from build123d import *

# Parameters (mm, degrees)
SKETCH1_R               = 18.5
BOSS_EXTRUDE1_DEPTH     = 60
SKETCH2_W               = 40
SKETCH2_H               = 37
BOSS_EXTRUDE2_DEPTH     = 58
SKETCH3_R               = 4
BOSS_EXTRUDE3_DEPTH     = 15
CUT_EXTRUDE1_DEPTH      = 125.282943319
CUT_EXTRUDE1_DEPTH_BACK = 58
SKETCH4_W               = 40
SKETCH4_H               = 10
SKETCH5_R               = 4
SKETCH5_R_2             = 2.25
BOSS_EXTRUDE4_DEPTH     = 1.5


with BuildPart() as part:
    # Sketch1 → Boss-Extrude1 (new body)
    with BuildSketch(Plane.XY):
        Circle(SKETCH1_R)
    extrude(amount=BOSS_EXTRUDE1_DEPTH)

    # Sketch2 → Boss-Extrude2 (add)
    with BuildSketch(Plane.XY.offset(60)):
        Rectangle(SKETCH2_W, SKETCH2_H)
    extrude(amount=BOSS_EXTRUDE2_DEPTH)

    # Sketch3 → Boss-Extrude3 (add)
    with BuildSketch(Plane(origin=(0, 18.5, 0), x_dir=(1, 0, 0), z_dir=(0, 1, 0))):
        with Locations(Location((0, -98, 0), (0, 0, 90))):
            Circle(SKETCH3_R)
    extrude(amount=BOSS_EXTRUDE3_DEPTH)

    # Sketch4 → Cut-Extrude1 (cut, two sides: drawn at the far end of the back side and taken through both)
    with BuildSketch(Plane.XY.offset(118).offset(-CUT_EXTRUDE1_DEPTH_BACK)):
        with Locations((0, -13.5)):
            Rectangle(SKETCH4_W, SKETCH4_H)
    extrude(amount=CUT_EXTRUDE1_DEPTH + CUT_EXTRUDE1_DEPTH_BACK, mode=Mode.SUBTRACT)

    # Sketch5 → Boss-Extrude4 (add)
    # profile 1 of 4: a face of its own
    with BuildSketch(Plane(origin=(0, 18.5, 0), x_dir=(1, 0, 0), z_dir=(0, 1, 0))):
        with Locations(Location((14, -69, 0), (0, 0, 90))):
            Circle(SKETCH5_R)
        with Locations(Location((14, -69, 0), (0, 0, 270))):
            Circle(SKETCH5_R_2, mode=Mode.SUBTRACT)
    # profile 2 of 4: a face of its own
    with BuildSketch(Plane(origin=(0, 18.5, 0), x_dir=(1, 0, 0), z_dir=(0, 1, 0))):
        with Locations(Location((14, -109, 0), (0, 0, 90))):
            Circle(SKETCH5_R)
        with Locations(Location((14, -109, 0), (0, 0, 270))):
            Circle(SKETCH5_R_2, mode=Mode.SUBTRACT)
    # profile 3 of 4: a face of its own
    with BuildSketch(Plane(origin=(0, 18.5, 0), x_dir=(1, 0, 0), z_dir=(0, 1, 0))):
        with Locations(Location((-14, -109, 0), (0, 0, 90))):
            Circle(SKETCH5_R)
        with Locations(Location((-14, -109, 0), (0, 0, 90))):
            Circle(SKETCH5_R_2, mode=Mode.SUBTRACT)
    # profile 4 of 4: a face of its own
    with BuildSketch(Plane(origin=(0, 18.5, 0), x_dir=(1, 0, 0), z_dir=(0, 1, 0))):
        with Locations(Location((-14, -69, 0), (0, 0, 90))):
            Circle(SKETCH5_R)
        with Locations(Location((-14, -69, 0), (0, 0, 90))):
            Circle(SKETCH5_R_2, mode=Mode.SUBTRACT)
    extrude(amount=BOSS_EXTRUDE4_DEPTH)


solid = part.part
The model under review builds one solid part; all positions refer to its coordinate system, in mm. A direction names the side the tool comes from. Give positions to 0.01 mm unless a question says otherwise; leave off trailing zeros. Loops run counter-clockwise (first coordinate to the right, second up) from the corner with the lowest first, then second, coordinate; pieces in that order, holes last. Notation, with made-up numbers: (53, -10.75) -> (57, -10.75) arc R33 cw to (57, 17.25) -> close; hole circle Ø11 at (36.25, 14). An arc over 180 degrees is marked (long way). Answer as a JSON object with one key per item and string values. Group by question number.
Q1. Draft analysis for pull direction X (two halves, no side actions). For faces 1 (the cylindrical face through (-4.01, -18.06, 29.58)), 2 (the cylindrical face through (-11.804, 19.24, 69.488)), 3 (the cylindrical face through (11.804, 19.24, 68.512)), 4 (the flat face through (0, 33.5, 98)), state which applies: pulls with the +X half, pulls with the -X half, needs draft (parallel to the pull), parting line crosses it, or undercut.
Q2. Wall thickness on line 1 along X through (y, z) = (19.2, 69); line 2 along Z through (x, y) = (-14, 19.5); line 3 along Y through (x, z) = (9.5, 113): over which ranges is each line inside the solid? List them lowest first.
Q3. Take a section at D-D (z = 98). Write out the cut boundary in (x, y), plus the area to 3 significant figures.
Q4. Take a section at B-B (y = -4.5). Write out the cut boundary in (x, z), plus the area to 3 significant figures.
Q5. Take a section at A-A (z = 69). Write out the cut boundary in (x, y).
Q6. Tool access review of faces 5 (the flat face through (-14, 18.5, 109)), 6 (the flat face through (16, 20, 67)), 7 (the flat face through (0, -8.5, 89)): name each direction out of +Z, -Z, +X, -X, +Y, -Y from which nothing blocks a thin tool from reaching the whole face with its end or side.
Q7. Take a section at C-C (x = -2). Write out the cut boundary in (y, z).
Q8. Insertion check: pin 1 (6.5 mm diameter, centred on x = -14.5, z = 67, fed in from +Y); pin 2 (5 mm diameter, centred on x = -14, z = 109, fed in from -Y); pin 3 (10 mm diameter, centred on x = 13, y = -6, fed in from -Z); pin 4 (1.5 mm diameter, centred on x = -6, z = 65.5, fed in from +Y). Each pin has a flat end and moves straight along its axis. Give the tip position at first contact, or say it passes through.
Answer below:
{
 "1": {"face 1": "parting line crosses it", "face 2": "undercut", "face 3": "undercut", "face 4": "needs draft"},
 "2": {"line 1": "x = -18 to -16.25, -11.75 to -10, 10 to 11.75, 16.25 to 18", "line 2": "z = 65 to 66.75, 71.25 to 73, 105 to 106.75, 111.25 to 113", "line 3": "y = -8.5 to 18.5"},
 "3": {"outline": "(-20, -8.5) -> (20, -8.5) -> (20, 18.5) -> (4, 18.5) -> (4, 33.5) -> (-4, 33.5) -> (-4, 18.5) -> (-20, 18.5) -> close", "area": "1,200 mm2"},
 "4": {"outline": "(-20, 60) -> (-17.94, 60) -> (-17.94, 0) -> (17.94, 0) -> (17.94, 60) -> (20, 60) -> (20, 118) -> (-20, 118) -> close", "area": "4,470 mm2"},
 "5": {"outline": "(-20, -8.5) -> (20, -8.5) -> (20, 18.5) -> (18, 18.5) -> (18, 20) -> (16.25, 20) -> (16.25, 18.5) -> (11.75, 18.5) -> (11.75, 20) -> (10, 20) -> (10, 18.5) -> (-10, 18.5) -> (-10, 20) -> (-11.75, 20) -> (-11.75, 18.5) -> (-16.25, 18.5) -> (-16.25, 20) -> (-18, 20) -> (-18, 18.5) -> (-20, 18.5) -> close"},
 "6": {"face 5": "+Y", "face 6": "+Z, -Z, +X, -X, +Y", "face 7": "+Z, +X, -X, -Y"},
 "7": {"outline": "(-18.39, 0) -> (18.39, 0) -> (18.39, 60) -> (18.5, 60) -> (18.5, 94.54) -> (33.5, 94.54) -> (33.5, 101.46) -> (18.5, 101.46) -> (18.5, 118) -> (-8.5, 118) -> (-8.5, 60) -> (-18.39, 60) -> close"},
 "8": {"pin 1": "stops at y = 20", "pin 2": "stops at y = -8.5", "pin 3": "stops at z = 0", "pin 4": "stops at y = 18.5"}
}
